The listing builds one solid part. Answer for the finished solid, in the listing's coordinates (mm). Face numbers are marked on the shaded views. A direction names the side the tool comes from. Give positions to 0.01 mm unless a question says otherwise; leave off trailing zeros. Write each loop counter-clockwise with the first axis right and the second up, starting at its lowest first coordinate (ties: lowest second). Pieces come first, ordered by that corner, then holes. Notation, with made-up numbers: M -12.5,-34 L 23.5,-34 A20 cw 23.5,-13 Z; hole C 15.5,-35.75 d11. An arc over 180 degrees is marked long. Answer as a JSON object with one key per item and string values.
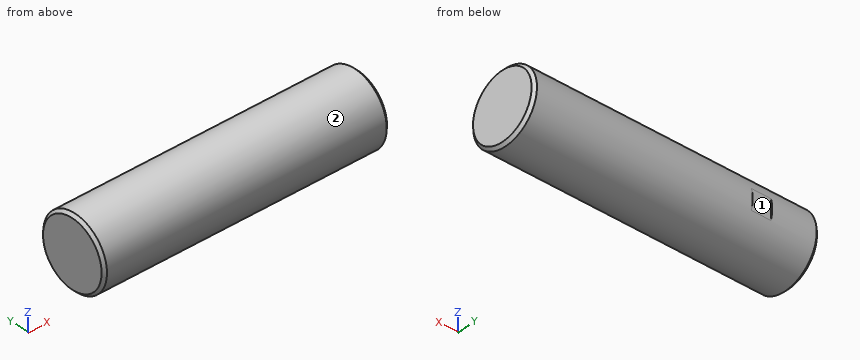
```python
from build123d import *

# Parameters (mm, degrees)
SKETCH2_R               = 3.175
BOSS_EXTRUDE1_DEPTH     = 25.4
CHAMFER1_SIZE           = 0.254
SKETCH3_W               = 1.733713748
SKETCH3_H               = 3.25599899
CUT_EXTRUDE1_DEPTH      = 4.175
CUT_EXTRUDE1_DEPTH_BACK = 4.175


with BuildPart() as part:
    # Sketch2 → Boss-Extrude1 (new body)
    with BuildSketch(Plane(origin=(0, 0, 0), x_dir=(0, 0, -1), z_dir=(1, 0, 0))):
        Circle(SKETCH2_R)
    extrude(amount=BOSS_EXTRUDE1_DEPTH)

    # Chamfer1
    chamfer1_edges = [part.edges().sort_by_distance(p)[0] for p in [
        (0, 0, 3.175),
        (25.4, 0, 3.175),
    ]]
    chamfer(chamfer1_edges, length=CHAMFER1_SIZE)

    # Sketch3 → Cut-Extrude1 (cut, two sides)
    with BuildSketch(Plane.XY) as cut_extrude1_sk:
        with Locations((5.08, 4.675999495)):
            Rectangle(SKETCH3_W, SKETCH3_H)
    extrude(amount=CUT_EXTRUDE1_DEPTH, mode=Mode.SUBTRACT)
    extrude(cut_extrude1_sk.sketch, amount=-CUT_EXTRUDE1_DEPTH_BACK, mode=Mode.SUBTRACT)


solid = part.part
```
1. Consider line 1 along Z through (x, y) = (12.5, -1.25); line 2 along Y through (x, z) = (19.75, 2.25). Determine where each line is inside the solid, lowest interval first.
Verdict:
{"line 1": "z = -2.92 to 2.92", "line 2": "y = -2.24 to 2.24"}
2. A flat-ended cylindrical pin translates along its axis: pin 1 (1.4 mm diameter, centred on x = 5, z = 0.5, fed in from +Y). Find the tip coordinate at first contact, or state that the pin passes through.
Verdict:
{"pin 1": "stops at y = 3.05"}
3. A cutting plane is placed at A-A, the plane x = 22.5. Give the vertices of the cut face in (y, z) (3 decimals).
Verdict:
{"outline": "C 0,0 d6.35"}
4. For the marked faces 1 and 2, determine the directions among +Z, -Z, +X, -X, +Y, -Y from which every point of the face is accessible in a straight line to the end or side of a thin tool.
Verdict:
{"face 1": "+Z, -Z, +Y", "face 2": "+X, -X"}
